Part model, mm, in its own coordinate system. A direction names the side the tool comes from. Give positions to 0.01 mm unless a question says otherwise; leave off trailing zeros. Order: outer loops, then holes, each group sorted by start corner. A loop starts at its lowest first (then second) coordinate and runs counter-clockwise, first axis right, second up. Notation, with made-up numbers: M -4,-33 L 42,-33 A19 ccw 42,3 Z; hole C -26.5,65.25 d1. An arc over 180 degrees is marked long. One line per question, with ' | ' between items.
```python
from build123d import *

# Parameters (mm, degrees)
F0_W     = 90.249106
F0_H     = 52.73592
F0_W_2   = 18.122312
F0_H_2   = 24.46512
F1_DEPTH = 12.7
F2_W     = 90.249106
F2_H     = 52.73592
F2_R     = 7.305338
F2_W_2   = 18.122312
F2_H_2   = 24.46512
F3_DEPTH = 12.7
F4_R     = 5.08


with BuildPart() as f1:
    # F0 (on Front) → F1 (new body, symmetric)
    with BuildSketch(Plane.XZ):
        Rectangle(F0_W, F0_H)
        Rectangle(F0_W_2, F0_H_2, mode=Mode.SUBTRACT)
    extrude(amount=F1_DEPTH, both=True)

    # F2 (on face) → F3 (join, symmetric)
    with BuildSketch(Plane.XZ.offset(12.7)):
        Rectangle(F2_W, F2_H)
        with Locations((-29.901814, 7.520759)):
            Circle(F2_R, mode=Mode.SUBTRACT)
        Rectangle(F2_W_2, F2_H_2, mode=Mode.SUBTRACT)
    extrude(amount=F3_DEPTH, both=True)

    # F4
    f4_edges = [f1.edges().sort_by_distance(p)[0] for p in [
        (-45.124553, -6.35, 26.36796),
        (-45.124553, 12.7, 0),
        (-45.124553, -6.35, -26.36796),
        (-45.124553, -25.4, 0),
    ]]
    fillet(f4_edges, radius=F4_R)


solid = f1.part
```
1. Slice it at C-C on y = -4.5. Give the cut face in (x, z).
Worked out:
outline: M -45.12,-21.29 A5.08 ccw -40.04,-26.37 L 45.12,-26.37 L 45.12,26.37 L -40.04,26.37 A5.08 ccw -45.12,21.29 Z; hole M -9.06,-12.23 L 9.06,-12.23 L 9.06,12.23 L -9.06,12.23 Z
2. Tool access for faces 1 (the flat face through (9.061, -7, 0)), 2 (the flat face through (-30, -12.7, 8)), 3 (the flat face through (-45.125, -7, 0)): list every direction of +Z, -Z, +X, -X, +Y, -Y with a clear straight run to the whole face (end or side of a thin tool).
Worked out:
face 1: +Y, -Y | face 2: -Y | face 3: +Z, -Z, -X, +Y, -Y
3. Mould opens along X. For faces 4 (the flat face through (45.125, -7, 0)), 5 (the flat face through (2, -7, 26.368)), 6 (the flat face through (0, -7, -12.233)), 7 (the flat face through (-9.061, -7, 0)) say: released by +X, released by -X, zero draft, split by the parting line, or undercut.
Worked out:
face 4: released by +X | face 5: zero draft | face 6: undercut | face 7: undercut
4. Drop a flat-ended pin along its axis: pin 1 (11.5 mm diameter, centred on x = -27.5, z = 6, fed in from -Y). Give the stop position or say it passes through.
Worked out:
pin 1: stops at y = -25.4
5. Probe L1, parallel to Z at x = -4.5, y = -5; L2, parallel to X at y = 4.5, z = -3.5; L3, parallel to X at y = -18, z = 10. List the from-to ranges inside material, lowest first. Write a range as from..to.
Worked out:
L1: z = -26.37..-12.23, 12.23..26.37 | L2: x = -45.12..-9.06, 9.06..45.12 | L3: x = -45.12..-36.77, -23.03..-9.06, 9.06..45.12
6. Slice it at A-A on z = -1. Give the cut face in (x, y), then the cut area to 3 significant figures.
Worked out:
outline: M -45.12,-20.32 A5.08 ccw -40.04,-25.4 L -9.06,-25.4 L -9.06,12.7 L -40.04,12.7 A5.08 ccw -45.12,7.62 Z; M 9.06,-25.4 L 45.12,-25.4 L 45.12,12.7 L 9.06,12.7 Z | area: 2,740 mm2
7. Slice it at D-D on y = -17.5. Give the cut face in (x, z), then the cut area to 3 significant figures.
Worked out:
outline: M -45.12,-21.29 A5.08 ccw -40.04,-26.37 L 45.12,-26.37 L 45.12,26.37 L -40.04,26.37 A5.08 ccw -45.12,21.29 Z; hole C -29.9,7.52 d14.61; hole M -9.06,-12.23 L 9.06,-12.23 L 9.06,12.23 L -9.06,12.23 Z | area: 4,140 mm2
8. Slice it at B-B on x = 1.5. Give the cut face in (y, z).
Worked out:
outline: M -25.4,-26.37 L 12.7,-26.37 L 12.7,-12.23 L -25.4,-12.23 Z; M -25.4,12.23 L 12.7,12.23 L 12.7,26.37 L -25.4,26.37 Z
